```python
from build123d import *

# Parameters (mm, degrees)
F1_DEPTH = 9


with BuildPart() as f1:
    # F0 (on Top) → F1 (new body)
    with BuildSketch(Plane.XY):
        with BuildLine():
            ThreePointArc((-14.697093, 2.999245), (-14.528747, 3.730348), (-14.324058, 4.45212))
            Line((-14.324058, 4.45212), (-16.261224, 4.9495))
            Line((-16.261224, 4.9495), (-16.634259, 3.496625))
            Line((-16.634259, 3.496625), (-14.697093, 2.999245))
        make_face()
        with BuildLine():
            ThreePointArc((-13.489474, 6.560037), (-13.1446, 7.226305), (-12.766844, 7.874497))
            Line((-12.766844, 7.874497), (-14.519457, 8.838004))
            Line((-14.519457, 8.838004), (-15.242088, 7.523544))
            Line((-15.242088, 7.523544), (-13.489474, 6.560037))
        make_face()
        with BuildLine():
            ThreePointArc((-11.434263, 9.708637), (-10.934529, 10.268207), (-10.407442, 10.80209))
            Line((-10.407442, 10.80209), (-11.86538, 12.171184))
            Line((-11.86538, 12.171184), (-12.8922, 11.077731))
            Line((-12.8922, 11.077731), (-11.434263, 9.708637))
        make_face()
        with BuildLine():
            ThreePointArc((-8.660595, 12.247208), (-8.037402, 12.664919), (-7.394103, 13.050948))
            Line((-7.394103, 13.050948), (-8.465757, 14.739604))
            Line((-8.465757, 14.739604), (-9.732248, 13.935864))
            Line((-9.732248, 13.935864), (-8.660595, 12.247208))
        make_face()
        with BuildLine():
            ThreePointArc((-14.981238, -0.75), (-15, 0), (-14.981238, 0.75))
            Line((-14.981238, 0.75), (-16.981238, 0.75))
            Line((-16.981238, 0.75), (-16.981238, -0.75))
            Line((-16.981238, -0.75), (-14.981238, -0.75))
        make_face()
        with BuildLine():
            Line((-16.261224, -4.9495), (-14.324058, -4.45212))
            ThreePointArc((-14.324058, -4.45212), (-14.528747, -3.730348), (-14.697093, -2.999245))
            Line((-14.697093, -2.999245), (-16.634259, -3.496625))
            Line((-16.634259, -3.496625), (-16.261224, -4.9495))
        make_face()
        with BuildLine():
            Line((-14.519457, -8.838004), (-12.766844, -7.874497))
            ThreePointArc((-12.766844, -7.874497), (-13.1446, -7.226305), (-13.489474, -6.560037))
            Line((-13.489474, -6.560037), (-15.242088, -7.523544))
            Line((-15.242088, -7.523544), (-14.519457, -8.838004))
        make_face()
        with BuildLine():
            ThreePointArc((14.957107, -1.133561), (14.989273, -0.567186), (15, 0))
            ThreePointArc((15, 0), (14.989273, 0.567186), (14.957107, 1.133561))
            ThreePointArc((14.957107, 1.133561), (14.881721, 1.879999), (14.769107, 2.621733))
            ThreePointArc((14.769107, 2.621733), (14.528747, 3.730348), (14.205296, 4.817629))
            ThreePointArc((14.205296, 4.817629), (13.946647, 5.521868), (13.65311, 6.212294))
            ThreePointArc((13.65311, 6.212294), (13.1446, 7.226305), (12.560915, 8.198988))
            ThreePointArc((12.560915, 8.198988), (12.135255, 8.816779), (11.679237, 9.412514))
            ThreePointArc((11.679237, 9.412514), (10.934529, 10.268207), (10.127286, 11.065174))
            ThreePointArc((10.127286, 11.065174), (9.56136, 11.557699), (8.971516, 12.02131))
            ThreePointArc((8.971516, 12.02131), (8.037402, 12.664919), (7.057321, 13.236095))
            ThreePointArc((7.057321, 13.236095), (6.386689, 13.572406), (5.700081, 13.874764))
            ThreePointArc((5.700081, 13.874764), (4.635255, 14.265848), (3.54392, 14.575343))
            ThreePointArc((3.54392, 14.575343), (2.81072, 14.734309), (2.070489, 14.856415))
            ThreePointArc((2.070489, 14.856415), (0.941858, 14.970401), (-0.19216, 14.998769))
            ThreePointArc((-0.19216, 14.998769), (-0.941858, 14.970401), (-1.6892, 14.904583))
            ThreePointArc((-1.6892, 14.904583), (-2.81072, 14.734309), (-3.916165, 14.479767))
            ThreePointArc((-3.916165, 14.479767), (-4.635255, 14.265848), (-5.34275, 14.016242))
            ThreePointArc((-5.34275, 14.016242), (-6.386689, 13.572406), (-7.394103, 13.050948))
            ThreePointArc((-7.394103, 13.050948), (-8.037402, 12.664919), (-8.660595, 12.247208))
            ThreePointArc((-8.660595, 12.247208), (-9.56136, 11.557699), (-10.407442, 10.80209))
            ThreePointArc((-10.407442, 10.80209), (-10.934529, 10.268207), (-11.434263, 9.708637))
            ThreePointArc((-11.434263, 9.708637), (-12.135255, 8.816779), (-12.766844, 7.874497))
            ThreePointArc((-12.766844, 7.874497), (-13.1446, 7.226305), (-13.489474, 6.560037))
            ThreePointArc((-13.489474, 6.560037), (-13.946647, 5.521868), (-14.324058, 4.45212))
            ThreePointArc((-14.324058, 4.45212), (-14.528747, 3.730348), (-14.697093, 2.999245))
            ThreePointArc((-14.697093, 2.999245), (-14.881721, 1.879999), (-14.981238, 0.75))
            ThreePointArc((-14.981238, 0.75), (-15, 0), (-14.981238, -0.75))
            ThreePointArc((-14.981238, -0.75), (-14.881721, -1.879999), (-14.697093, -2.999245))
            ThreePointArc((-14.697093, -2.999245), (-14.528747, -3.730348), (-14.324058, -4.45212))
            ThreePointArc((-14.324058, -4.45212), (-13.946647, -5.521868), (-13.489474, -6.560037))
            ThreePointArc((-13.489474, -6.560037), (-13.1446, -7.226305), (-12.766844, -7.874497))
            ThreePointArc((-12.766844, -7.874497), (-12.135255, -8.816779), (-11.434263, -9.708637))
            ThreePointArc((-11.434263, -9.708637), (-10.934529, -10.268207), (-10.407442, -10.80209))
            ThreePointArc((-10.407442, -10.80209), (-9.56136, -11.557699), (-8.660595, -12.247208))
            ThreePointArc((-8.660595, -12.247208), (-8.037402, -12.664919), (-7.394103, -13.050948))
            ThreePointArc((-7.394103, -13.050948), (-6.386689, -13.572406), (-5.34275, -14.016242))
            ThreePointArc((-5.34275, -14.016242), (-4.635255, -14.265848), (-3.916165, -14.479767))
            ThreePointArc((-3.916165, -14.479767), (-2.81072, -14.734309), (-1.6892, -14.904583))
            ThreePointArc((-1.6892, -14.904583), (-0.941858, -14.970401), (-0.19216, -14.998769))
            ThreePointArc((-0.19216, -14.998769), (0.941858, -14.970401), (2.070489, -14.856415))
            ThreePointArc((2.070489, -14.856415), (2.81072, -14.734309), (3.54392, -14.575343))
            ThreePointArc((3.54392, -14.575343), (4.635255, -14.265848), (5.700081, -13.874764))
            ThreePointArc((5.700081, -13.874764), (6.386689, -13.572406), (7.057321, -13.236095))
            ThreePointArc((7.057321, -13.236095), (8.037402, -12.664919), (8.971516, -12.02131))
            ThreePointArc((8.971516, -12.02131), (9.56136, -11.557699), (10.127286, -11.065174))
            ThreePointArc((10.127286, -11.065174), (10.934529, -10.268207), (11.679237, -9.412514))
            ThreePointArc((11.679237, -9.412514), (12.135255, -8.816779), (12.560915, -8.198988))
            ThreePointArc((12.560915, -8.198988), (13.1446, -7.226305), (13.65311, -6.212294))
            ThreePointArc((13.65311, -6.212294), (13.946647, -5.521868), (14.205296, -4.817629))
            ThreePointArc((14.205296, -4.817629), (14.528747, -3.730348), (14.769107, -2.621733))
            ThreePointArc((14.769107, -2.621733), (14.881721, -1.879999), (14.957107, -1.133561))
        make_face()
        with BuildLine():
            ThreePointArc((-2.284732, -2.45), (-3.35, 0), (-2.284732, 2.45))
            Line((-2.284732, 2.45), (2.284732, 2.45))
            ThreePointArc((2.284732, 2.45), (3.35, 0), (2.284732, -2.45))
            Line((2.284732, -2.45), (-2.284732, -2.45))
        make_face(mode=Mode.SUBTRACT)
        with BuildLine():
            Line((-11.86538, -12.171184), (-10.407442, -10.80209))
            ThreePointArc((-10.407442, -10.80209), (-10.934529, -10.268207), (-11.434263, -9.708637))
            Line((-11.434263, -9.708637), (-12.8922, -11.077731))
            Line((-12.8922, -11.077731), (-11.86538, -12.171184))
        make_face()
        with BuildLine():
            Line((-8.465757, -14.739604), (-7.394103, -13.050948))
            ThreePointArc((-7.394103, -13.050948), (-8.037402, -12.664919), (-8.660595, -12.247208))
            Line((-8.660595, -12.247208), (-9.732248, -13.935864))
            Line((-9.732248, -13.935864), (-8.465757, -14.739604))
        make_face()
        with BuildLine():
            ThreePointArc((-5.34275, 14.016242), (-4.635255, 14.265848), (-3.916165, 14.479767))
            Line((-3.916165, 14.479767), (-4.534199, 16.38188))
            Line((-4.534199, 16.38188), (-5.960784, 15.918355))
            Line((-5.960784, 15.918355), (-5.34275, 14.016242))
        make_face()
        with BuildLine():
            ThreePointArc((-1.6892, 14.904583), (-0.941858, 14.970401), (-0.19216, 14.998769))
            Line((-0.19216, 14.998769), (-0.317741, 16.994823))
            Line((-0.317741, 16.994823), (-1.814781, 16.900637))
            Line((-1.814781, 16.900637), (-1.6892, 14.904583))
        make_face()
        with BuildLine():
            ThreePointArc((2.070489, 14.856415), (2.81072, 14.734309), (3.54392, 14.575343))
            Line((3.54392, 14.575343), (3.918682, 16.539918))
            Line((3.918682, 16.539918), (2.445251, 16.82099))
            Line((2.445251, 16.82099), (2.070489, 14.856415))
        make_face()
        with BuildLine():
            ThreePointArc((5.700081, 13.874764), (6.386689, 13.572406), (7.057321, 13.236095))
            Line((7.057321, 13.236095), (7.90888, 15.045749))
            Line((7.90888, 15.045749), (6.551639, 15.684418))
            Line((6.551639, 15.684418), (5.700081, 13.874764))
        make_face()
        with BuildLine():
            ThreePointArc((8.971516, 12.02131), (9.56136, 11.557699), (10.127286, 11.065174))
            Line((10.127286, 11.065174), (11.402134, 12.606201))
            Line((11.402134, 12.606201), (10.246364, 13.562337))
            Line((10.246364, 13.562337), (8.971516, 12.02131))
        make_face()
        with BuildLine():
            ThreePointArc((11.679237, 9.412514), (12.135255, 8.816779), (12.560915, 8.198988))
            Line((12.560915, 8.198988), (14.178949, 9.374559))
            Line((14.178949, 9.374559), (13.297271, 10.588084))
            Line((13.297271, 10.588084), (11.679237, 9.412514))
        make_face()
        with BuildLine():
            ThreePointArc((13.65311, 6.212294), (13.946647, 5.521868), (14.205296, 4.817629))
            Line((14.205296, 4.817629), (16.064849, 5.553878))
            Line((16.064849, 5.553878), (15.512663, 6.948543))
            Line((15.512663, 6.948543), (13.65311, 6.212294))
        make_face()
        with BuildLine():
            ThreePointArc((14.769107, 2.621733), (14.881721, 1.879999), (14.957107, 1.133561))
            Line((14.957107, 1.133561), (16.941336, 1.384227))
            Line((16.941336, 1.384227), (16.753336, 2.8724))
            Line((16.753336, 2.8724), (14.769107, 2.621733))
        make_face()
        with BuildLine():
            Line((16.941336, -1.384227), (14.957107, -1.133561))
            ThreePointArc((14.957107, -1.133561), (14.881721, -1.879999), (14.769107, -2.621733))
            Line((14.769107, -2.621733), (16.753336, -2.8724))
            Line((16.753336, -2.8724), (16.941336, -1.384227))
        make_face()
        with BuildLine():
            Line((16.064849, -5.553878), (14.205296, -4.817629))
            ThreePointArc((14.205296, -4.817629), (13.946647, -5.521868), (13.65311, -6.212294))
            Line((13.65311, -6.212294), (15.512663, -6.948543))
            Line((15.512663, -6.948543), (16.064849, -5.553878))
        make_face()
        with BuildLine():
            Line((14.178949, -9.374559), (12.560915, -8.198988))
            ThreePointArc((12.560915, -8.198988), (12.135255, -8.816779), (11.679237, -9.412514))
            Line((11.679237, -9.412514), (13.297271, -10.588084))
            Line((13.297271, -10.588084), (14.178949, -9.374559))
        make_face()
        with BuildLine():
            Line((11.402134, -12.606201), (10.127286, -11.065174))
            ThreePointArc((10.127286, -11.065174), (9.56136, -11.557699), (8.971516, -12.02131))
            Line((8.971516, -12.02131), (10.246364, -13.562337))
            Line((10.246364, -13.562337), (11.402134, -12.606201))
        make_face()
        with BuildLine():
            Line((7.90888, -15.045749), (7.057321, -13.236095))
            ThreePointArc((7.057321, -13.236095), (6.386689, -13.572406), (5.700081, -13.874764))
            Line((5.700081, -13.874764), (6.551639, -15.684418))
            Line((6.551639, -15.684418), (7.90888, -15.045749))
        make_face()
        with BuildLine():
            Line((3.918682, -16.539918), (3.54392, -14.575343))
            ThreePointArc((3.54392, -14.575343), (2.81072, -14.734309), (2.070489, -14.856415))
            Line((2.070489, -14.856415), (2.445251, -16.82099))
            Line((2.445251, -16.82099), (3.918682, -16.539918))
        make_face()
        with BuildLine():
            Line((-0.317741, -16.994823), (-0.19216, -14.998769))
            ThreePointArc((-0.19216, -14.998769), (-0.941858, -14.970401), (-1.6892, -14.904583))
            Line((-1.6892, -14.904583), (-1.814781, -16.900637))
            Line((-1.814781, -16.900637), (-0.317741, -16.994823))
        make_face()
        with BuildLine():
            Line((-4.534199, -16.38188), (-3.916165, -14.479767))
            ThreePointArc((-3.916165, -14.479767), (-4.635255, -14.265848), (-5.34275, -14.016242))
            Line((-5.34275, -14.016242), (-5.960784, -15.918355))
            Line((-5.960784, -15.918355), (-4.534199, -16.38188))
        make_face()
    extrude(amount=F1_DEPTH)


solid = f1.part
```
Part model, mm, in its own coordinate system. A direction names the side the tool comes from. Give positions to 0.01 mm unless a question says otherwise; leave off trailing zeros. Write each loop counter-clockwise with the first axis right and the second up, starting at its lowest first coordinate (ties: lowest second). Pieces come first, ordered by that corner, then holes. Notation, with made-up numbers: (-26.5, -1) -> (32.5, -1) arc R19 cw to (32.5, 27) -> close; hole circle Ø3 at (-1.5, -11.75). An arc over 180 degrees is marked (long way). Put each result on its own line as item: value. Start each with the question number.
Item 1: Pin check, flat tips, straight feed: pin 1 Ø1.6 at (x, z) = (-16, 4) entering from +Y; pin 2 Ø2 at (y, z) = (10.5, 7) entering from -X; pin 3 Ø2 at (x, z) = (-16, 5) entering from -Y. Stop position of each tip, or through.
Item 2: Cut at C-C (x = -8). List the corners of the cut face in (y, z), then the cut area to 3 significant figures.
Item 3: Cut at B-B (x = 5). List the corners of the cut face in (y, z), then the cut area to 3 significant figures.
Item 4: Wall check: L1, parallel to Y at x = -12, z = 8.25; L2, parallel to Y at x = -9, z = 7.75; L3, parallel to Y at x = 0, z = 1.75. Give the ranges that are in metal, low to high. Write a range as [from, to].
Item 5: Cut at A-A (y = -2). List the corners of the cut face in (x, z).
Item 6: Pull direction Y, two halves, no side cores. Call faces 1 (the face through (-12, 9, 4)), 2 (the face through (-6.37, 13.58, 4.44)), 3 (the face through (-0.254, 15.983, 4.437)), 4 (the face through (-11.15, -11.5, 4.44)): pulls with the +Y half, pulls with the -Y half, needs draft (parallel to the pull), parting line crosses it, or undercut.
Item 7: Which spindle directions (+Z, -Z, +X, -X, +Y, -Y) get a long thin tool onto all of the face, cutting with end or side? Do faces 5 (the face through (10.945, 10.257, 4.437)), 6 (the face through (-1.077, -16.947, 4.437)), 7 (the face through (9.618, 12.803, 4.437)), 8 (the face through (-4, 0, 0)), 9 (the face through (-15.68, 3.25, 4.44)). Say none if no direction does.
Answer list:
1. pin 1: stops at y = 7.6
1. pin 2: stops at x = -12.89
1. pin 3: stops at y = -7.96
2. outline: (-14.01, 0) -> (14.01, 0) -> (14.01, 9) -> (-14.01, 9) -> close
2. area: 252 mm2
3. outline: (-14.14, 0) -> (14.14, 0) -> (14.14, 9) -> (-14.14, 9) -> close
3. area: 255 mm2
4. L1: y = [-12.03, -10.24], [-9, 9], [10.24, 12.03]
4. L2: y = [-14.4, -12.78], [-12, 12], [12.78, 14.4]
4. L3: y = [-15, -2.45], [2.45, 15]
5. outline: (-14.87, 0) -> (-2.69, 0) -> (-2.69, 9) -> (-14.87, 9) -> close; (2.69, 0) -> (16.86, 0) -> (16.86, 9) -> (2.69, 9) -> close
6. face 1: undercut
6. face 2: undercut
6. face 3: pulls with the +Y half
6. face 4: pulls with the -Y half
7. face 5: +Z, -Z
7. face 6: +Z, -Z, -X, -Y
7. face 7: +Z, -Z, +Y
7. face 8: -Z, +X, -X, +Y, -Y
7. face 9: +Z, -Z, -X
